Geometry: see drawing. Coordinates: mm, zero at the bounding-box minimum. Round coordinates to 2 decimals unless told otherwise and drop trailing zeros. Write each loop counter-clockwise with the first axis right and the second up, starting at its lowest first coordinate (ties: lowest second). Pieces come first, ordered by that corner, then holes.
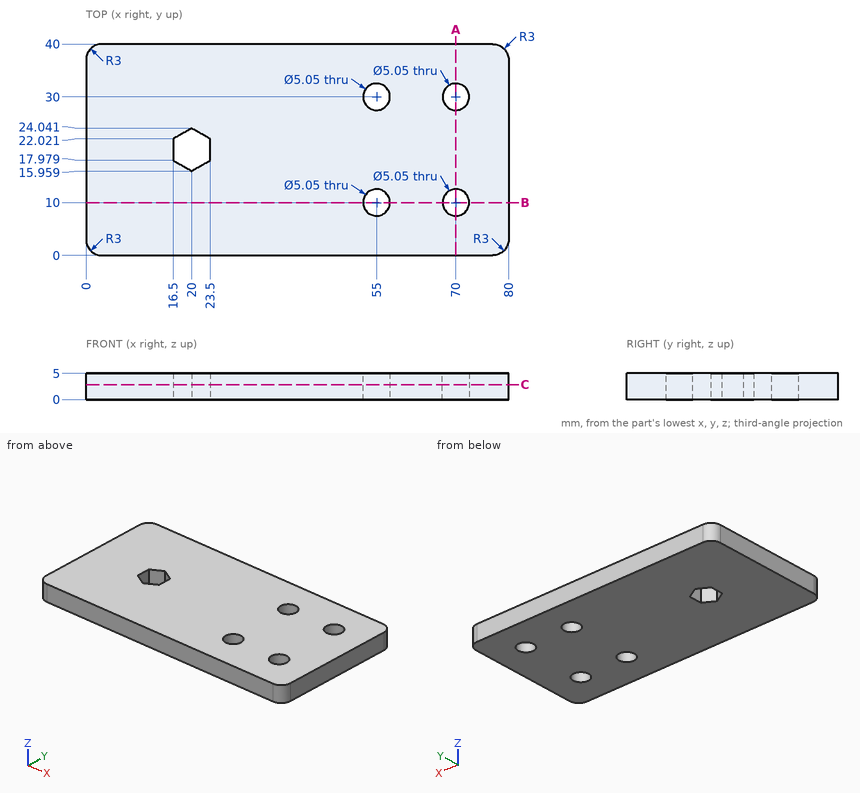
1) Section query B-B on y = 10. Return the cut outline in (x, z) (1 decimal).
Taken from the geometry:
outline: (0, 0) - (52.5, 0) - (52.5, 5) - (0, 5) - close; (57.5, 0) - (67.5, 0) - (67.5, 5) - (57.5, 5) - close; (72.5, 0) - (80, 0) - (80, 5) - (72.5, 5) - close
2) Material intervals for line 1 (Y direction, x = 70, z = 2.9) (1 decimal); line 2 (X direction, y = 12, z = 3.2); line 3 (X direction, y = 11.5, z = 4.4), sorted ascending.
Taken from the geometry:
line 1: y = 0 to 7.5, 12.5 to 27.5, 32.5 to 40
line 2: x = 0 to 53.46, 56.54 to 68.46, 71.54 to 80
line 3: x = 0 to 52.97, 57.03 to 67.97, 72.03 to 80
3) Section query C-C on z = 2.85. State how many separate pieces and enclosed holes the cut face has, then the cut area to 3 significant figures.
Taken from the geometry:
separate pieces: 1
enclosed holes: 5
area: 3,070 mm2
4) Section query A-A on x = 70. Return the cut outline in (y, z) (1 decimal).
Taken from the geometry:
outline: (0, 0) - (7.5, 0) - (7.5, 5) - (0, 5) - close; (12.5, 0) - (27.5, 0) - (27.5, 5) - (12.5, 5) - close; (32.5, 0) - (40, 0) - (40, 5) - (32.5, 5) - close
